Verification items for this drawing (mm, ordinates from the low corner). A direction names the side the tool comes from. Give positions to 0.01 mm unless a question says otherwise; leave off trailing zeros. Order: outer loops, then holes, each group sorted by start corner. A loop starts at its lowest first (then second) coordinate and runs counter-clockwise, first axis right, second up. Notation, with made-up numbers: M 20,51 L 53,51 A16 ccw 53,66 Z; hole C 77.5,0.5 d6. An arc over 180 degrees is marked long. Answer as a JSON object with one key per item and string values.
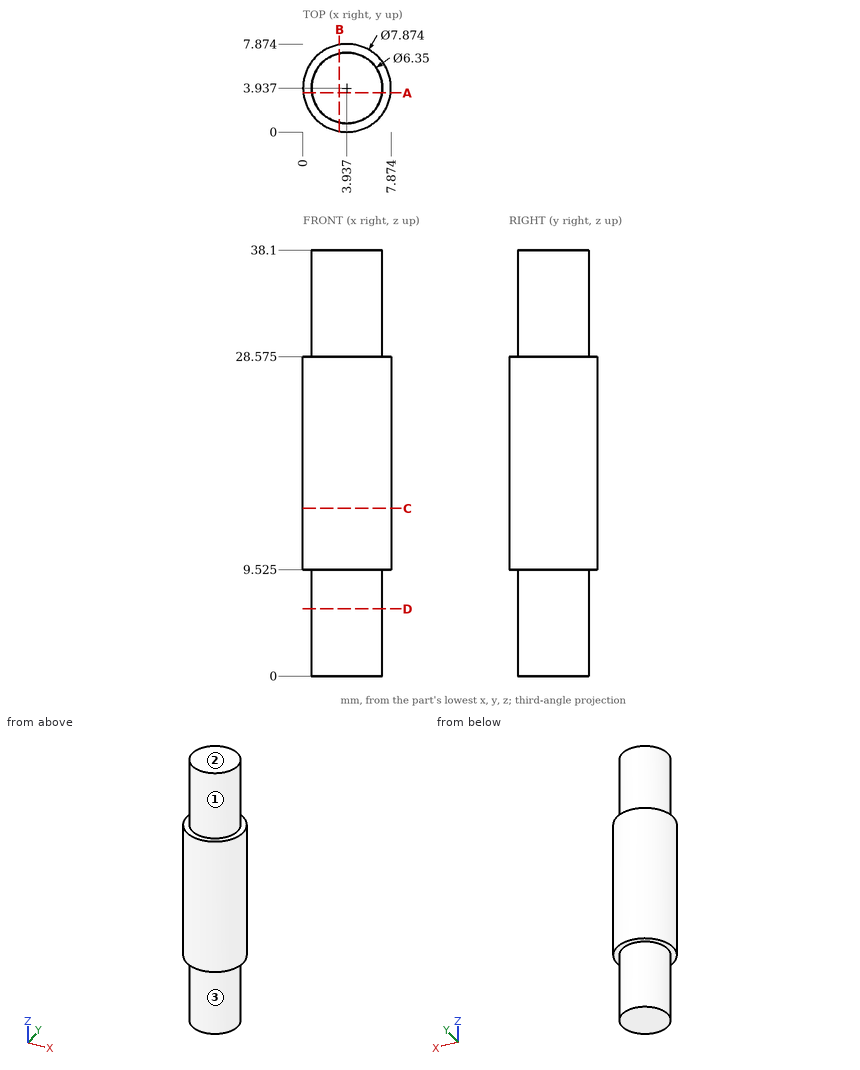
Q1. Section check C-C on z = 15. Record the cut outline in (x, y), then the cut area to 3 significant figures.
Resolved:
{"outline": "C 3.94,3.94 d7.87", "area": "48.7 mm²"}
Q2. Section check B-B on x = 3.25. Record the cut outline in (y, z) (3 decimals).
Resolved:
{"outline": "M 0.06,9.525 L 0.837,9.525 L 0.837,0 L 7.037,0 L 7.037,9.525 L 7.814,9.525 L 7.814,28.575 L 7.037,28.575 L 7.037,38.1 L 0.837,38.1 L 0.837,28.575 L 0.06,28.575 Z"}
Q3. Material ranges on L1, parallel to X at y = 3.75, z = 16; L2, parallel to X at y = 7, z = 15; L3, parallel to Z at x = 2.5, y = 0.5 (3 decimals), recorded low to high.
Resolved:
{"L1": "x = 0 to 7.87", "L2": "x = 1.46 to 6.41", "L3": "z = 9.525 to 28.575"}
Q4. Section check A-A on y = 3.5. Record the cut outline in (x, z) (3 decimals), then the cut area to 3 significant figures.
Resolved:
{"outline": "M 0.024,9.525 L 0.792,9.525 L 0.792,0 L 7.082,0 L 7.082,9.525 L 7.85,9.525 L 7.85,28.575 L 7.082,28.575 L 7.082,38.1 L 0.792,38.1 L 0.792,28.575 L 0.024,28.575 Z", "area": "269 mm²"}
Q5. Section check D-D on z = 6. Record the cut outline in (x, y) (3 decimals), then the cut area to 3 significant figures.
Resolved:
{"outline": "C 3.937,3.937 d6.35", "area": "31.7 mm²"}
Q6. Gauge pin test, flat ends, axial feed: pin 1 Ø1.5 at (x, z) = (6, 15) entering from +Y; pin 2 Ø1 at (x, z) = (5.5, 27) entering from -Y. Record the tip position at first contact, or that the pin passes through.
Resolved:
{"pin 1": "stops at y = 7.65", "pin 2": "stops at y = 0.15"}
Q7. Tool access check on the marked faces 1, 2 and 3. Record the directions out of +Z, -Z, +X, -X, +Y, -Y that give a thin tool (end or side, any length) a straight path to the whole face; none if there is none.
Resolved:
{"face 1": "+Z", "face 2": "+Z, +X, -X, +Y, -Y", "face 3": "-Z"}
